Geometry: final body of the model. Coordinates: model frame, mm. A direction names the side the tool comes from. Give positions to 0.01 mm unless a question says otherwise; leave off trailing zeros. Write each loop counter-clockwise with the first axis right and the second up, starting at its lowest first coordinate (ties: lowest second). Pieces come first, ordered by that corner, then holes. Notation, with made-up numbers: (-8, -29) - (22, -29) arc R23 ccw to (22, -12) - close; hole circle Ø5 at (-7.75, 30). An arc over 180 degrees is marked (long way). Use CSV: the item, a comma, the result in double quotes. Start each with the question number.
(1) Line query: probe 1 along Y at (x, z) = (47, 2.4); probe 2 along Y at (x, z) = (59.5, 4.55); probe 3 along X at (y, z) = (16, 2.3). Output: solid intervals per line, ascending. Write a range as [from, to].
(2) Section D-D on z = 5.15. Count the separate pieces of the cut face and the enclosed holes in it, and give its area (3 significant figures).
(3) First-contact query: pin 1 Ø3 at (y, z) = (19, 2) entering from -X. Flat tip, straight axial feed; report the tip coordinate or a pass-through.
(4) Section A-A on x = 62. Output: boundary loops of the cut face in (y, z).
(5) Section C-C on x = 70.5. Output: boundary loops of the cut face in (y, z).
(6) Reachability of faces 4 (the flat face through (59, 87.366, 3)), 5 (the flat face through (78.484, 77, 3)) from +Z, -Z, +X, -X, +Y, -Y: full face, straight path, thin tool, end or side. Return the list, or none.
(7) Draft query along X for faces 1 (the cylindrical face through (40.252, 32.483, 2.958)), 2 (the flat face through (56, 48, 6)), 3 (the flat face through (28.81, 53.43, 2.96)). Return one class per face: released by +X, released by -X, zero draft, split by the parting line, or undercut.
(8) Section B-B on y = 18. Output: boundary loops of the cut face in (x, z), and give its area (3 significant figures).
from build123d import *

# Parameters (mm, degrees)
MODEL_R                  = 1.8
MODEL_R_2                = 4.1
MODEL_W                  = 20.368459162
MODEL_H                  = 6.9
MODEL_W_2                = 10.4
MODEL_H_2                = 6.8
RESSALTO_EXTRUS_O1_DEPTH = 6


with BuildPart() as part:
    # Model → Ressalto-extrusão1 (new body)
    with BuildSketch(Plane.XY):
        Polygon((86.284167453, 87.365706057), (30.284167453, 87.365706057), (30.284167453, 54.904792152), (27.284167453, 51.904792152), (27.284167453, 42.926619963), (30.284167453, 39.926619963), (30.284167453, 7.465706057), (86.284167453, 7.465706057), align=None)
        with Locations((39.284167453, 30.965706057)):
            Circle(MODEL_R, mode=Mode.SUBTRACT)
        with Locations((81.284167453, 24.915706057)):
            Circle(MODEL_R, mode=Mode.SUBTRACT)
        with Locations((81.284167453, 69.915706057)):
            Circle(MODEL_R, mode=Mode.SUBTRACT)
        with Locations((39.284167453, 63.865706057)):
            Circle(MODEL_R, mode=Mode.SUBTRACT)
        with Locations((35.284167453, 47.415706057)):
            Circle(MODEL_R_2, mode=Mode.SUBTRACT)
        with Locations((66.417398963, 32.115706057)):
            Rectangle(MODEL_W, MODEL_H, mode=Mode.SUBTRACT)
        with Locations((44.284167453, 17.465706057)):
            Rectangle(MODEL_W_2, MODEL_H_2, mode=Mode.SUBTRACT)
        with Locations((44.284167453, 77.365706057)):
            Rectangle(MODEL_W_2, MODEL_H_2, mode=Mode.SUBTRACT)
        with Locations((66.417398963, 62.715706057)):
            Rectangle(MODEL_W, MODEL_H, mode=Mode.SUBTRACT)
        with Locations((73.284167453, 17.465706057)):
            Rectangle(MODEL_W_2, MODEL_H_2, mode=Mode.SUBTRACT)
        with Locations((73.284167453, 77.365706057)):
            Rectangle(MODEL_W_2, MODEL_H_2, mode=Mode.SUBTRACT)
    extrude(amount=RESSALTO_EXTRUS_O1_DEPTH)


solid = part.part
Check values:
1,probe 1,"y = [7.47, 14.07], [20.87, 73.97], [80.77, 87.37]"
1,probe 2,"y = [7.47, 28.67], [35.57, 59.27], [66.17, 87.37]"
1,probe 3,"x = [30.28, 39.08], [49.48, 68.08], [78.48, 86.28]"
2,separate pieces,"1"
2,enclosed holes,"11"
2,area,"3,850 mm²"
3,pin 1,"stops at x = 30.28"
4,outline,"(7.47, 0) - (28.67, 0) - (28.67, 6) - (7.47, 6) - close; (35.57, 0) - (59.27, 0) - (59.27, 6) - (35.57, 6) - close; (66.17, 0) - (87.37, 0) - (87.37, 6) - (66.17, 6) - close"
5,outline,"(7.47, 0) - (14.07, 0) - (14.07, 6) - (7.47, 6) - close; (20.87, 0) - (28.67, 0) - (28.67, 6) - (20.87, 6) - close; (35.57, 0) - (59.27, 0) - (59.27, 6) - (35.57, 6) - close; (66.17, 0) - (73.97, 0) - (73.97, 6) - (66.17, 6) - close; (80.77, 0) - (87.37, 0) - (87.37, 6) - (80.77, 6) - close"
6,face 4,"+Z, -Z, +X, -X, +Y"
6,face 5,"+Z, -Z"
7,face 1,"undercut"
7,face 2,"zero draft"
7,face 3,"released by -X"
8,outline,"(30.28, 0) - (39.08, 0) - (39.08, 6) - (30.28, 6) - close; (49.48, 0) - (68.08, 0) - (68.08, 6) - (49.48, 6) - close; (78.48, 0) - (86.28, 0) - (86.28, 6) - (78.48, 6) - close"
8,area,"211 mm²"
